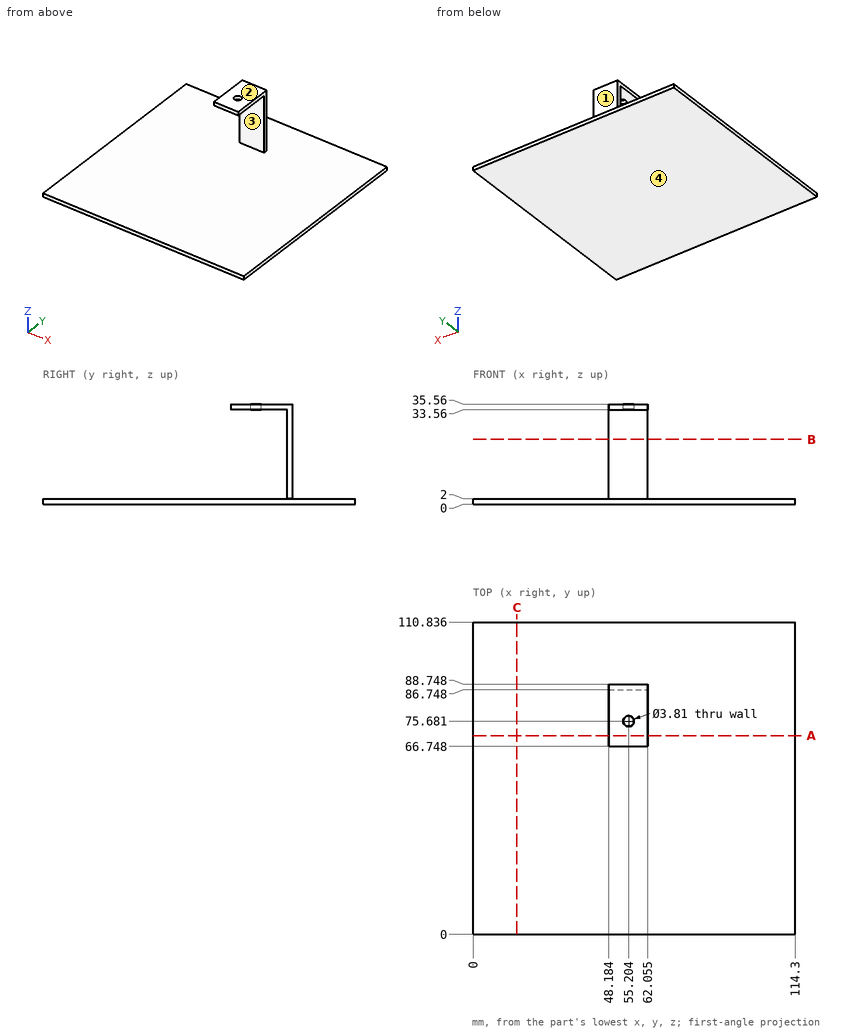
Study the drawing (mm; zero at the part's minimum x, y, z) and answer. Give positions to 0.01 mm unless a question says otherwise; leave off trailing zeros. Order: outer loops, then holes, each group sorted by start corner. A loop starts at its lowest first (then second) coordinate and runs counter-clockwise, first axis right, second up. Notation, with made-up numbers: (-14.75, -20.5) - (6.25, -20.5) arc R38 cw to (6.25, 17.5) - close; hole circle Ø6 at (0, -39.5). An arc over 180 degrees is marked (long way). Use one line per item in the form item = value. Start each with the question number.
(1) A cutting plane is placed at B-B, the plane z = 23. Write down the section's boundary in (x, y) (1 decimal).
(2) Consider line 1 (Z direction, x = 105, y = 16). Determine where the line is inside the solid, lowest interval first. Write a range as from..to.
(3) A cutting plane is placed at C-C, the plane x = 15.5. Write down the section's boundary in (y, z).
(4) The mould has two halves that part along Z. Classify the marked faces 1, 2, 3 and 4: released by +Z, released by -Z, zero draft, split by the parting line, or undercut.
(5) A cutting plane is placed at A-A, the plane y = 70.5. Write down the section's boundary in (x, z) (1 decimal).
(6) Flat-ended cylindrical pins translate along their axes: pin 1 Ø4 at (y, z) = (88, 10) entering from -X; pin 2 Ø5 at (x, y) = (77.5, 66.5) entering from +Z; pin 3 Ø11 at (x, z) = (56, 14) entering from -Y. Find the tip coordinate at first contact, or state that the pin passes through.
Ans:
q1.outline = (48.2, 86.7) - (62.1, 86.7) - (62.1, 88.7) - (48.2, 88.7) - close
q2.line_1 = 0..2
q3.outline = (0, 0) - (110.84, 0) - (110.84, 2) - (0, 2) - close
q4.face_1 = zero draft
q4.face_2 = released by +Z
q4.face_3 = undercut
q4.face_4 = released by -Z
q5.outline = (0, 0) - (114.3, 0) - (114.3, 2) - (0, 2) - close; (48.2, 33.6) - (62.1, 33.6) - (62.1, 35.6) - (48.2, 35.6) - close
q6.pin_1 = 48.18
q6.pin_2 = 2
q6.pin_3 = 86.75
